```python
from build123d import *

# Parameters (mm, degrees)
F2_DEPTH = 12
F3_W     = 28.1
F3_H     = 76.4
F7_DEPTH = 3
F4_W     = 28.1
F4_H     = 76.4
F8_DEPTH = 3
F9_D     = 5
F10_D    = 5


with BuildPart() as f2:
    # F1 (on Top) → F2 (new body)
    with BuildSketch(Plane.XY):
        Polygon((-35.0215807557, 39.4811810493), (-63.1215807557, 39.4811810493), (-63.1215807557, 36.4811810493), (-56.2715807557, 36.4811810493), (-56.2715807557, 31.6811810493), (-38.0215807557, 31.6811810493), (-38.0215807557, 9.0811810493), (-56.2715807557, 9.0811810493), (-56.2715807557, 4.2811810493), (-63.1215807557, 4.2811810493), (-63.1215807557, -1.7188189507), (-56.2715807557, -1.7188189507), (-56.2715807557, -6.5188189507), (-38.0215807557, -6.5188189507), (-38.0215807557, -29.1188189507), (-56.2715807557, -29.1188189507), (-56.2715807557, -33.9188189507), (-63.1215807557, -33.9188189507), (-63.1215807557, -36.9188189507), (-35.0215807557, -36.9188189507), align=None)
    extrude(amount=F2_DEPTH)

    # F3 (on face) → F7 (join)
    with BuildSketch(Plane.XY.offset(12)):
        with Locations((-49.0715807557, 1.2811810493)):
            Rectangle(F3_W, F3_H)
    extrude(amount=F7_DEPTH)

    # F4 (on face) → F8 (join)
    with BuildSketch(Plane(origin=(0, 0, 0), x_dir=(1, 0, 0), z_dir=(0, 0, -1))):
        with Locations((-49.0715807557, -1.2811810493)):
            Rectangle(F4_W, F4_H)
    extrude(amount=F8_DEPTH)

    # F9 (through all)
    with Locations(Plane(origin=(-38.0215807557, 0, 0), x_dir=(0, -1, 0), z_dir=(-1, 0, 0))):
        with Locations((-25.6811810493, 6)):
            Hole(F9_D / 2)

    # F10 (through all)
    with Locations(Plane(origin=(-38.0215807557, 0, 0), x_dir=(0, -1, 0), z_dir=(-1, 0, 0))):
        with Locations((23.1188189507, 6)):
            Hole(F10_D / 2)


solid = f2.part
```
Could you check a few things on this model? Use its own coordinates, in mm. A direction names the side the tool comes from. Give positions to 0.01 mm unless a question says otherwise; leave off trailing zeros. Loops run counter-clockwise (first coordinate to the right, second up) from the corner with the lowest first, then second, coordinate; pieces in that order, holes last. Notation, with made-up numbers: (-36.5, 5.25) - (-32.5, 5.25) arc R11 cw to (-32.5, 12.25) - close; hole circle Ø11 at (74, -5.75). An arc over 180 degrees is marked (long way). Answer in a Markdown table with one row per item. Add a question column.
Q1. If we section it at C-C (y = 27.5): List the corners of the cut face in (x, z) for me, plus the area to 3 significant figures.
Q2. Which directions (+Z, -Z, +X, -X, +Y, -Y) give clear straight access to the entire face, cutting with the end or side of a thin tool? Please do faces 4 (the face through (-36.501, -21.775, 8.108)), 5 (the face through (-60, -33.919, 6)).
Q3. For pin 1 (1.4 mm diameter, centred on y = -3.5, z = 7, fed in from -X); pin 2 (6 mm diameter, centred on y = 23, z = 7.5, fed in from -X), each with a flat end and sliding along its axis, tell me the tip position at first contact or that it passes through.
Q4. We'd pull the mould along Z, two halves only. Please class faces 1 (the face through (-63.122, 2, 8)), 2 (the face through (-49, 2, 15)), 3 (the face through (-56.272, -4, 6)): +Z half, -Z half, draft (parallel to the pull), parting line (faces both ways), or undercut.
Q5. If we section it at A-A (z = 6): List the corners of the cut face in (x, y) for me.
Q6. Please list where these lines run through material, in increasing order: L1, parallel to Y at x = -48.25, z = 6.25; L2, parallel to Y at x = -57.25, z = 6; L3, parallel to Z at x = -41, y = 25. Write a range as from..to.
Q7. If we section it at B-B (x = -58.5): List the corners of the cut face in (y, z) for me.
Q8. If we section it at D-D (z = 1): List the corners of the cut face in (x, y) for me, plus the area to 3 significant figures.
The answers:
| question | item | result |
|---|---|---|
| 1 | outline | (-63.12, -3) - (-35.02, -3) - (-35.02, 4.28) - (-38.02, 4.28) - (-38.02, 0) - (-63.12, 0) - close; (-63.12, 12) - (-38.02, 12) - (-38.02, 7.72) - (-35.02, 7.72) - (-35.02, 15) - (-63.12, 15) - close |
| 1 | area | 194 mm^2 |
| 2 | face 4 | +X, -X |
| 2 | face 5 | -X |
| 3 | pin 1 | stops at x = -56.27 |
| 3 | pin 2 | stops at x = -38.02 |
| 4 | face 1 | draft |
| 4 | face 2 | +Z half |
| 4 | face 3 | undercut |
| 5 | outline | (-63.12, -36.92) - (-35.02, -36.92) - (-35.02, -25.62) - (-38.02, -25.62) - (-38.02, -29.12) - (-56.27, -29.12) - (-56.27, -33.92) - (-63.12, -33.92) - close; (-63.12, -1.72) - (-56.27, -1.72) - (-56.27, -6.52) - (-38.02, -6.52) - (-38.02, -20.62) - (-35.02, -20.62) - (-35.02, 23.18) - (-38.02, 23.18) - (-38.02, 9.08) - (-56.27, 9.08) - (-56.27, 4.28) - (-63.12, 4.28) - close; (-63.12, 36.48) - (-56.27, 36.48) - (-56.27, 31.68) - (-38.02, 31.68) - (-38.02, 28.18) - (-35.02, 28.18) - (-35.02, 39.48) - (-63.12, 39.48) - close |
| 6 | L1 | y = -36.92..-29.12, -6.52..9.08, 31.68..39.48 |
| 6 | L2 | y = -36.92..-33.92, -1.72..4.28, 36.48..39.48 |
| 6 | L3 | z = -3..0, 12..15 |
| 7 | outline | (-36.92, -3) - (39.48, -3) - (39.48, 15) - (-36.92, 15) - close; hole (-33.92, 0) - (-1.72, 0) - (-1.72, 12) - (-33.92, 12) - close; hole (4.28, 0) - (36.48, 0) - (36.48, 12) - (4.28, 12) - close |
| 8 | outline | (-63.12, -36.92) - (-35.02, -36.92) - (-35.02, 39.48) - (-63.12, 39.48) - (-63.12, 36.48) - (-56.27, 36.48) - (-56.27, 31.68) - (-38.02, 31.68) - (-38.02, 9.08) - (-56.27, 9.08) - (-56.27, 4.28) - (-63.12, 4.28) - (-63.12, -1.72) - (-56.27, -1.72) - (-56.27, -6.52) - (-38.02, -6.52) - (-38.02, -29.12) - (-56.27, -29.12) - (-56.27, -33.92) - (-63.12, -33.92) - close |
| 8 | area | 881 mm^2 |
